Work out the finished part from the listing and answer in its coordinate system (mm). Face numbers are marked on the shaded views. A direction names the side the tool comes from. Give positions to 0.01 mm unless a question says otherwise; leave off trailing zeros. Order: outer loops, then holes, each group sorted by start corner. A loop starts at its lowest first (then second) coordinate and runs counter-clockwise, first axis right, second up. Notation, with made-up numbers: (26, 14) - (66, 14) arc R11 ccw to (66, 25) - close; hole circle Ø7 at (1, -27). An arc over 180 degrees is marked (long way). Return JSON: item names as keys, results as strings. Group by question number.
Autodesk Fusion 360 part; units mm, degrees
sketch "Sketch1" plane through (0, 0, 0) normal (0, 0, 1) x (1, 0, 0) in component "Light Braccket"
  line L0 (0, 0) -> (-25, 0)
  line L1 (-25, 0) -> (-25, 25)
  line L2 (-25, 25) -> (0, 25)
  line L3 (0, 25) -> (0, 0)
  dimension "d1" = 25
  dimension "d2" = 25
extrude "Extrude1" add sketch "Sketch1" along normal blind 25 in component "Light Braccket"
sketch "Sketch2" plane through (0, 0, 0) normal (0, -1, 0) x (1, 0, 0) in component "Light Braccket"
  line L0 (-25, 0) -> (0, 0)
  line L1 (0, 0) -> (0, 25)
  line L2 (0, 25) -> (-25, 25)
  line L3 (-25, 25) -> (-25, 0)
  line L4 (-0.3536, 0) -> (-2.9142, 1.0607)
  line L5 (-0.3536, 0) -> (0.9236, 0) construction
  line L6 (-2.9142, 1.0607) -> (-0.9142, 1.0607)
  line L7 (-0.9142, 1.0607) -> (-0.9142, 16.0607)
  line L8 (-0.9142, 18.8102) -> (-15.9142, 18.8102) construction
  line L9 (-8.4142, 18.8102) -> (-8.4142, -0.114) construction
  line L10 (-16.4749, 0) -> (-13.9142, 1.0607)
  line L11 (-13.9142, 1.0607) -> (-15.9142, 1.0607)
  line L12 (-15.9142, 1.0607) -> (-15.9142, 16.0607)
  line L13 (-0.9142, 16.0607) -> (-15.9142, 16.0607)
  dimension "d14" = 15
extrude "Extrude2" cut sketch "Sketch2" against normal blind 40 contours L0 L4 L6 L7 L10 L11 L12 L13 in component "Light Braccket"
sketch "Sketch3" plane through (0, 0, 0) normal (0, -1, 0) x (1, 0, 0) in component "Light Braccket"
  line L0 (-16.4749, 0) -> (-13.9142, 1.0607)
  line L1 (-13.9142, 1.0607) -> (-15.9142, 1.0607)
  line L2 (-15.9142, 1.0607) -> (-15.9142, 16.0607)
  line L3 (-15.9142, 16.0607) -> (-0.9142, 16.0607)
  line L4 (-0.9142, 16.0607) -> (-0.9142, 1.0607)
  line L5 (-0.9142, 1.0607) -> (-2.9142, 1.0607)
  line L6 (-2.9142, 1.0607) -> (-0.3536, 0)
  line L7 (-0.3536, 0) -> (0, 0)
  line L8 (0, 0) -> (0, 25)
  line L9 (0, 25) -> (-25, 25)
  line L10 (-25, 25) -> (-25, 0)
  line L11 (-25, 0) -> (-16.4749, 0)
  line L12 (-25, 25) -> (0, 25)
  line L13 (0, 25) -> (0, 19)
  line L14 (0, 19) -> (-25, 19)
  line L15 (-25, 19) -> (-25, 25)
extrude "Extrude3" cut sketch "Sketch3" against normal blind 39 contours L8 L9 L10 L12 L13 L14 L15 in component "Light Braccket"
sketch "Sketch4" plane through (0, 0, 0) normal (0, -1, 0) x (1, 0, 0) in component "Light Braccket"
  line L0 (0, 19) -> (-25, 19)
  line L1 (-25, 19) -> (-25, 0)
  line L2 (-25, 0) -> (-16.4749, 0)
  line L3 (-16.4749, 0) -> (-13.9142, 1.0607)
  line L4 (-13.9142, 1.0607) -> (-15.9142, 1.0607)
  line L5 (-15.9142, 1.0607) -> (-15.9142, 16.0607)
  line L6 (-15.9142, 16.0607) -> (-0.9142, 16.0607)
  line L7 (-0.9142, 16.0607) -> (-0.9142, 1.0607)
  line L8 (-0.9142, 1.0607) -> (-2.9142, 1.0607)
  line L9 (-2.9142, 1.0607) -> (-0.3536, 0)
  line L10 (-0.3536, 0) -> (0, 0)
  line L11 (0, 0) -> (0, 19)
  line L12 (-25, 0) -> (-25, 6.6)
  line L13 (-25, 6.6) -> (-21.8712, 3.4712)
  line L14 (-25, 6.6) -> (-20.5752, 6.6) construction
  line L15 (-21.8712, 3.4712) -> (-21.8712, 8)
  line L16 (-21.8712, 8) -> (-20.3712, 8)
  line L17 (-20.3712, 8) -> (-20.3712, 0)
  line L18 (-25, 0) -> (-20.3712, 0)
  line L19 (-25, 9.5) -> (0, 9.5) construction
  line L20 (-25, 12.4) -> (-21.8712, 15.5288)
  line L21 (-21.8712, 15.5288) -> (-21.8712, 11)
  line L22 (-20.3712, 11) -> (-20.3712, 19)
  line L23 (-21.8712, 11) -> (-20.3712, 11)
  line L24 (-25, 19) -> (-20.3712, 19)
  line L25 (-25, 19) -> (-25, 12.4)
  dimension "d19" = 6.6
  dimension "d20" = 45
  dimension "d21" = 1.5
extrude "Extrude4" cut sketch "Sketch4" against normal blind 33.5 contours L0 L1 L20 L21 L22 L23 L24 L25 | L1 L2 L12 L13 L15 L16 L17 L18 in component "Light Braccket"
sketch "Sketch1 (2)" plane through (0, 0, 0) normal (1, 0, 0) x (0, 1, 0)
  line L0 (25, 19) -> (0, 19)
  line L1 (0, 19) -> (0, 0)
  line L2 (0, 0) -> (25, 0)
  line L3 (25, 0) -> (25, 19)
extrude "Extrude5" add sketch "Sketch1 (2)" along normal blind 3 in component "Light Braccket"
fillet "Fillet2" radius 0.5 7 edges at (-8.6856, 0, 19) (-20.3712, 12.5, 19) (-8.6856, 25, 19) (3, 12.5, 19) (3, 0, 9.5) (3, 25, 9.5) (3, 12.5, 0) in component "Light Braccket"
component "Light Braccket" placed x (1, 0, 0) y (0, 1, 0) z (0, 0, 1) at (0, 0, 0)
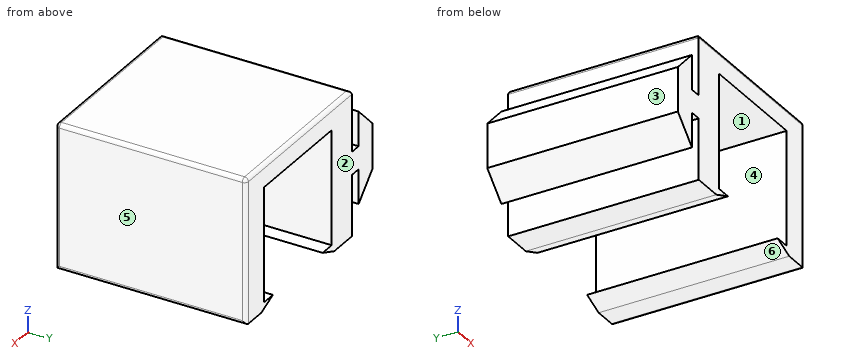
1. The part is cut by section A-A (z = 3). Give the vertices of the cut face in (x, y).
2. The part is cut by section D-D (y = 15.5). Give the vertices of the cut face in (x, z).
3. A tool of negligible diameter and unlimited length cuts with its end or side. For the marked faces 4, 5 and 6, from which of +Z, -Z, +X, -X, +Y, -Y can it reach the whole face along a straight path? Write none if from no direction.
4. The part is cut by section C-C (x = -11). Give the vertices of the cut face in (y, z), and give its area (3 significant figures).
5. Determine the mould class of the marked faces 1, 2 and 3 for opening direction X: released by +X, released by -X, zero draft, split by the parting line, or undercut.
6. Each of these flat-tipped pins is pushed along its axis until it touches: pin 1 (0.8 mm diameter, centred on x = -21, y = 12.5, fed in from +Z); pin 2 (8 mm diameter, centred on y = 14.5, z = 2.5, fed in from -X); pin 3 (6 mm diameter, centred on y = 8, z = 16.5, fed in from -X). Where does it stop, or does it pass through?
7. The part is cut by section B-B (z = 13.5). Give the vertices of the cut face in (x, y).
8. Consider probe 1 along X at (y, z) = (7, 12); probe 2 along X at (y, z) = (6.25, 15.75); probe 3 along X at (y, z) = (7.5, 15). Determine where each line is inside the solid, lowest interval first. Write a range as from..to.
Answers:
{
 "1": {"outline": "(-20.37, 0) - (-15.91, 0) - (-15.91, 25) - (-20.37, 25) - close; (-0.91, 0) - (2.5, 0) arc R0.5 ccw to (3, 0.5) - (3, 24.5) arc R0.5 ccw to (2.5, 25) - (-0.91, 25) - close"},
 "2": {"outline": "(-25, 6.6) - (-21.87, 3.47) - (-21.87, 8) - (-20.37, 8) - (-20.37, 0) - (-16.47, 0) - (-13.91, 1.06) - (-15.91, 1.06) - (-15.91, 16.06) - (-0.91, 16.06) - (-0.91, 1.06) - (-2.91, 1.06) - (-0.35, 0) - (2.5, 0) arc R0.5 ccw to (3, 0.5) - (3, 18.5) arc R0.5 ccw to (2.5, 19) - (-19.87, 19) arc R0.5 ccw to (-20.37, 18.5) - (-20.37, 11) - (-21.87, 11) - (-21.87, 15.53) - (-25, 12.4) - close"},
 "3": {"face 4": "+Y, -Y", "face 5": "+Z, -Z, +X, +Y, -Y", "face 6": "-Z, +Y, -Y"},
 "4": {"outline": "(0, 16.06) - (25, 16.06) - (25, 18.5) arc R0.5 ccw to (24.5, 19) - (0.5, 19) arc R0.5 ccw to (0, 18.5) - close", "area": "73.4 mm^2"},
 "5": {"face 1": "undercut", "face 2": "zero draft", "face 3": "released by -X"},
 "6": {"pin 1": "stops at z = 11", "pin 2": "stops at x = -24.9", "pin 3": "stops at x = -23.9"},
 "7": {"outline": "(-23.9, 0) - (-21.87, 0) - (-21.87, 25) - (-23.9, 25) - close; (-20.37, 0) - (-15.91, 0) - (-15.91, 25) - (-20.37, 25) - close; (-0.91, 0) - (2.5, 0) arc R0.5 ccw to (3, 0.5) - (3, 24.5) arc R0.5 ccw to (2.5, 25) - (-0.91, 25) - close"},
 "8": {"probe 1": "x = -25..-21.87, -20.37..-15.91, -0.91..3", "probe 2": "x = -20.37..-15.91, -0.91..3", "probe 3": "x = -22.4..-21.87, -20.37..-15.91, -0.91..3"}
}
